```python
from build123d import *

# Parameters (mm, degrees)
SKETCH1_R           = 3
SKETCH1_R_2         = 2.5000000000000004
BOSS_EXTRUDE1_DEPTH = 15
SKETCH2_R           = 5
SKETCH2_R_2         = 3.0000000000000004
BOSS_EXTRUDE2_DEPTH = 2.5
FILLET1_R           = 2.5
FILLET2_R           = 2.5


with BuildPart() as part:
    # Sketch1 → Boss-Extrude1 (new body)
    with BuildSketch(Plane(origin=(0, 0, 0), x_dir=(0, 0, -1), z_dir=(1, 0, 0))):
        Circle(SKETCH1_R)
        Circle(SKETCH1_R_2, mode=Mode.SUBTRACT)
    extrude(amount=BOSS_EXTRUDE1_DEPTH)

    # Sketch2 → Boss-Extrude2 (add)
    with BuildSketch(Plane(origin=(0, 0, 0), x_dir=(0, 0, -1), z_dir=(1, 0, 0))):
        Circle(SKETCH2_R)
        Circle(SKETCH2_R_2, mode=Mode.SUBTRACT)
    extrude(amount=BOSS_EXTRUDE2_DEPTH)

    # Fillet1
    # the kernel refuses this fillet: 2.5 mm, written as the material it adds along each edge
    with BuildSketch(Plane(origin=(2.5, 0, 0), x_dir=(0, 0, -1), z_dir=(0, -1, 0))) as fillet1_piece_1:
        with BuildLine():
            CenterArc((5.5, 2.449489742786441), FILLET1_R, 180, 78.4630409671995)
            Line((5.0000000000006395, 3.13216e-12), (4.990000000000652, -0.04898979485253419))
            ThreePointArc((4.990000000000652, -0.04898979485253419), (4.00000000000032, -0.04999999999999982), (3.0000000000000004, -0.04999999999999982))
            Line((3.0000000000000004, -0.04999999999999982), (2.9500000000000006, 0))
            Line((2.9500000000000006, 0), (2.95, 2.449489742786441))
            Line((2.95, 2.449489742786441), (3, 2.449489742786441))
        make_face()
    revolve(axis=Axis((2.5, 0, 0), (1, 0, 0)))

    # Fillet2
    fillet2_edges = [part.edges().sort_by_distance(p)[0] for p in [
        (2.5, 6.1e-16, 5),
    ]]
    fillet(fillet2_edges, radius=FILLET2_R)


solid = part.part
```
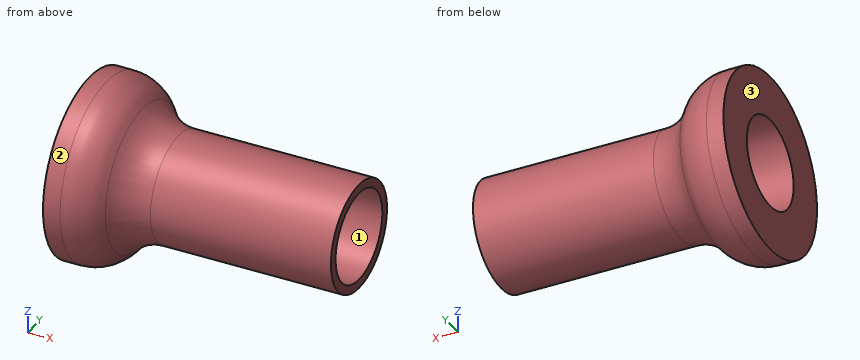
Geometry check sheet. Reference: the model listing, model coordinates, mm. Face numbers are marked on the shaded views. Give positions to 0.01 mm unless a question says otherwise; leave off trailing zeros. Write each loop counter-clockwise with the first axis right and the second up, starting at its lowest first coordinate (ties: lowest second). Pieces come first, ordered by that corner, then holes. Notation, with made-up numbers: (-2, 1.5) -> (32, 1.5) arc R21 cw to (32, 12.5) -> close; hole circle Ø6 at (52, -10). An arc over 180 degrees is marked (long way). Use one line per item in the form item = value.
Item 1: Sectioned sample at A-A on x = 5.5. Enter the section's corners in (y, z), plus the area to 3 significant figures.
Results list:
outline = circle Ø6 at (0, 0); hole circle Ø5 at (0, 0)
area = 8.64 mm2
Item 2: Depth check by flat-ended pin: pin 1 Ø6 at (x, y) = (5, 0) entering from -Z; pin 2 Ø3 at (x, y) = (4, -3) entering from +Z; pin 3 Ø6 at (y, z) = (0, 0) entering from -X; pin 4 Ø1 at (x, z) = (11.5, -0.5) entering from +Y. Enter the tip coordinate at first touch or a pass-through.
Results list:
pin_1 = -4.77
pin_2 = 3.65
pin_3 = 0
pin_4 = 3
Item 3: Mould release check, pull along Z, two halves, no side actions. Record for the marked faces 1, 2 and 3: released by +Z, released by -Z, zero draft, split by the parting line, or undercut.
Results list:
face_1 = undercut
face_2 = split by the parting line
face_3 = zero draft
Item 4: Scan lines: line 1 (Y direction, x = 9, z = 0); line 2 (Y direction, x = 2.5, z = -1.5); line 3 (Z direction, x = 5.75, y = -2.25). Record each from-to range of solid material in increasing order.
Results list:
line_1 = -3 to -2.5, 2.5 to 3
line_2 = -4.2 to -2, 2 to 4.2
line_3 = -1.98 to -1.09, 1.09 to 1.98
